Source: CAD feature listing. Evaluate the final solid. Frame: model axes, mm. A direction names the side the tool comes from. Give positions to 0.01 mm unless a question says otherwise; leave off trailing zeros. Loops run counter-clockwise (first coordinate to the right, second up) from the corner with the lowest first, then second, coordinate; pieces in that order, holes last. Notation, with made-up numbers: (46, -6.5) - (104, -6.5) arc R12 cw to (104, 13.5) - close; hole circle Ø6 at (38.5, -28). An arc over 180 degrees is marked (long way). Write each question's results on one line, items separated by ' | '. Start each with the question number.
(1) Contact query for flat-ended pins moving along their axis: pin 1 (1.5 mm diameter, centred on y = 4.5, z = 0, fed in from -X); pin 2 (1 mm diameter, centred on x = 43.5, z = -0.5, fed in from -Y); pin 3 (5 mm diameter, centred on x = 76, y = 3, fed in from -Z). Output: stop coordinate, or through.
(2) Reachability of faces 4 (the cylindrical face through (152.449, 2.385, 1.197)), 5 (the cylindrical face through (-0.97, -0.92, 1.81)) from +Z, -Z, +X, -X, +Y, -Y: full face, straight path, thin tool, end or side. Return the list, or none.
(3) Cut plane A-A on x = 9. Return the cut outline in (y, z), then the cut area to 3 significant figures.
(4) Material intervals for line 1 along Y through (x, z) = (65, -0.3); line 2 along Y through (x, z) = (54.5, -0.4); line 3 along X through (y, z) = (3.25, 0.65), sorted ascending. Write a range as [from, to].
(5) Pull-direction query (X, two-part tool) for faces 1 (the cylindrical face through (155.92, 10.97, 1.81)), 2 (the cylindrical face through (-0.97, 10.92, 1.81)), 3 (the cylindrical face through (2.551, 7.615, 1.197)); classes: pulls with the +X half, pulls with the -X half, needs draft (parallel to the pull), parting line crosses it, or undercut.
from build123d import *

# Parameters (mm, degrees)
F0_W         = 155
F0_H         = 10
F0_W_2       = 152.0637926605
F0_H_2       = 7.2836262298
F1_DEPTH     = 1.2
F2_W         = 159
F2_H         = 14
F2_W_2       = 155
F2_H_2       = 10
F2_W_3       = 152.0637926605
F2_H_3       = 7.2836262298
F3_DEPTH     = 1.2
F4_W         = 155
F4_H         = 1
F5_DEPTH     = 1.2
F6_R         = 3.6
F7_T1_DEPTH  = 160
F7_T3_DEPTH  = 0.0836262298
F7_T5_DEPTH  = 144.8637926605
F7_T10_ANGLE = 129.8047192326
F7_T13_ANGLE = 90
F7_T17_ANGLE = 129.8047192326
F7_T22_ANGLE = 129.8047192326
F7_T25_ANGLE = 90
F7_T27_ANGLE = 90
F7_T29_ANGLE = 90
F7_T33_ANGLE = 129.8047192326
F8_F1_R      = 0.5
F8_F2_R      = 0.5
F8_F3_R      = 0.5


# Not quite as in the source:
# - a fillet or chamfer that OpenCascade refuses, or shapes differently, is made with other operations: its cross-section is extruded or revolved along the edge and cut away or added


with BuildPart() as f1:
    # F0 (on Top) → F1 (new body)
    with BuildSketch(Plane.XY):
        with Locations((77.5, 5)):
            Rectangle(F0_W, F0_H)
        with Locations((77.5, 5)):
            Rectangle(F0_W_2, F0_H_2, mode=Mode.SUBTRACT)
    extrude(amount=F1_DEPTH)

    # F2 (on face) → F3 (join)
    with BuildSketch(Plane.XY.offset(1.2)):
        with Locations((77.5, 5)):
            Rectangle(F2_W, F2_H)
        with Locations((77.5, 5)):
            Rectangle(F2_W_2, F2_H_2, mode=Mode.SUBTRACT)
        with Locations((77.5, 5)):
            Rectangle(F2_W_2, F2_H_2)
        with Locations((77.5, 5)):
            Rectangle(F2_W_3, F2_H_3, mode=Mode.SUBTRACT)
    extrude(amount=F3_DEPTH)

    # F4 (on face) → F5 (join)
    with BuildSketch(Plane(origin=(0, 0, 0), x_dir=(1, 0, 0), z_dir=(0, 0, -1))):
        with Locations((77.5, 0.5)):
            Rectangle(F4_W, F4_H)
        Polygon((155, -1.3581868851), (155, 0), (0, 0), (0, -1.3581868851), (1.4681036697, -1.3581868851), (153.5318963303, -1.3581868851), align=None)
        Polygon((155, -10), (155, -8.6418131149), (153.5318963303, -8.6418131149), (1.4681036697, -8.6418131149), (0, -8.6418131149), (0, -10), align=None)
        with Locations((77.5, -10.5)):
            Rectangle(F4_W, F4_H)
    extrude(amount=F5_DEPTH)

    # F6
    f6_edges = [f1.edges().sort_by_distance(p)[0] for p in [
        (1.468104, 1.358187, 1.2),
        (1.468104, 8.641813, 1.2),
        (153.531896, 1.358187, 1.2),
        (153.531896, 8.641813, 1.2),
        (157, -2, 1.8),
        (157, 12, 1.8),
        (-2, 12, 1.8),
        (-2, -2, 1.8),
    ]]
    fillet(f6_edges, radius=F6_R)

    # F7: fillet of radius 1 on 16 edges, made by hand

    # F7_s2 → F7_t1 (cut)
    with BuildSketch(Plane.YZ.offset(-2.5)):
        with BuildLine():
            ThreePointArc((1.3581868851, -0.2), (1.0652936663, -0.9071067812), (0.3581868851, -1.2))
            Line((0.3581868851, -1.2), (1.3581868851, -1.2))
            Line((1.3581868851, -1.2), (1.3581868851, -0.2))
        make_face()
        with BuildLine():
            ThreePointArc((8.6418131149, -0.2), (8.9347063337, -0.9071067812), (9.6418131149, -1.2))
            Line((9.6418131149, -1.2), (8.6418131149, -1.2))
            Line((8.6418131149, -1.2), (8.6418131149, -0.2))
        make_face()
    extrude(amount=F7_T1_DEPTH, mode=Mode.SUBTRACT)

    # F7_s4 → F7_t3 (cut)
    with BuildSketch(Plane.XZ.offset(-5.0418131149)):
        with BuildLine():
            ThreePointArc((0.4681036697, 0), (1.1752104509, 0.2928932188), (1.4681036697, 1))
            Line((1.4681036697, 1), (1.4681036697, 0))
            Line((1.4681036697, 0), (0.4681036697, 0))
        make_face()
        with BuildLine():
            ThreePointArc((1.4681036697, 1.4), (1.1752104509, 2.1071067812), (0.4681036697, 2.4))
            Line((0.4681036697, 2.4), (1.4681036697, 2.4))
            Line((1.4681036697, 2.4), (1.4681036697, 1.4))
        make_face()
        with BuildLine():
            ThreePointArc((154.5318963303, 2.4), (153.8247895491, 2.1071067812), (153.5318963303, 1.4))
            Line((153.5318963303, 1.4), (153.5318963303, 2.4))
            Line((153.5318963303, 2.4), (154.5318963303, 2.4))
        make_face()
        with BuildLine():
            ThreePointArc((154.5318963303, 0), (153.8247895491, 0.2928932188), (153.5318963303, 1))
            Line((153.5318963303, 1), (153.5318963303, 0))
            Line((153.5318963303, 0), (154.5318963303, 0))
        make_face()
    extrude(amount=F7_T3_DEPTH, mode=Mode.SUBTRACT)

    # F7_s6 → F7_t5 (cut)
    with BuildSketch(Plane.YZ.offset(5.0681036697)):
        with BuildLine():
            ThreePointArc((1.3581868851, 1.4), (1.0652936663, 2.1071067812), (0.3581868851, 2.4))
            Line((0.3581868851, 2.4), (1.3581868851, 2.4))
            Line((1.3581868851, 2.4), (1.3581868851, 1.4))
        make_face()
        with BuildLine():
            ThreePointArc((8.6418131149, 1.4), (8.9347063337, 2.1071067812), (9.6418131149, 2.4))
            Line((9.6418131149, 2.4), (8.6418131149, 2.4))
            Line((8.6418131149, 2.4), (8.6418131149, 1.4))
        make_face()
    extrude(amount=F7_T5_DEPTH, mode=Mode.SUBTRACT)


with BuildPart() as f7_tool8:
    # F7_s9 → F7_t10 (revolve)
    with BuildSketch(Plane(origin=(0.5115194158, -0.4262532935, 0), x_dir=(0, 0, 1), z_dir=(0.7682307976, -0.6401729779, 0))):
        with BuildLine():
            ThreePointArc((0, -11.7177391291), (0.2928932188, -11.0106323479), (1, -10.7177391291))
            Line((1, -10.7177391291), (0, -10.7177391291))
            Line((0, -10.7177391291), (0, -11.7177391291))
        make_face()
    revolve(axis=Axis((5.0681036697, 5.0418131149, 0), (0, 0, 1)), revolution_arc=F7_T10_ANGLE)

    split(bisect_by=Plane.XZ.offset(-8.6418131149), keep=Keep.TOP)


with BuildPart() as f1_1:
    add(f1.part)

    # F7_t7: cut F7_tool8
    add(f7_tool8.part, mode=Mode.SUBTRACT)

    # F7_s12 → F7_t13 (revolve, cut)
    with BuildSketch(Plane.YZ.offset(5.0681036697)):
        with BuildLine():
            ThreePointArc((8.6418131149, 1.4), (8.9347063337, 2.1071067812), (9.6418131149, 2.4))
            Line((9.6418131149, 2.4), (8.6418131149, 2.4))
            Line((8.6418131149, 2.4), (8.6418131149, 1.4))
        make_face()
    revolve(axis=Axis((5.0681036697, 5.0418131149, 2.4), (0, 0, 1)), revolution_arc=F7_T13_ANGLE, mode=Mode.SUBTRACT)


with BuildPart() as f7_tool15:
    # F7_s16 → F7_t17 (revolve)
    with BuildSketch(Plane(origin=(90.9661571375, 75.8028393036, 0), x_dir=(0, 0, 1), z_dir=(-0.7682307976, -0.6401729779, 0))):
        with BuildLine():
            ThreePointArc((0, -87.5090724404), (0.2928932188, -88.2161792216), (1, -88.5090724404))
            Line((1, -88.5090724404), (0, -88.5090724404))
            Line((0, -88.5090724404), (0, -87.5090724404))
        make_face()
    revolve(axis=Axis((149.9318963303, 5.0418131149, 0), (0, 0, -1)), revolution_arc=F7_T17_ANGLE)

    split(bisect_by=Plane.XZ.offset(-8.6418131149), keep=Keep.TOP)


with BuildPart() as f1_2:
    add(f1_1.part)

    # F7_t14: cut F7_tool15
    add(f7_tool15.part, mode=Mode.SUBTRACT)


with BuildPart() as f7_tool20:
    # F7_s21 → F7_t22 (revolve)
    with BuildSketch(Plane.XZ.offset(-4.9581868851)):
        with BuildLine():
            ThreePointArc((0.4681036697, 0), (1.1752104509, 0.2928932188), (1.4681036697, 1))
            Line((1.4681036697, 1), (1.4681036697, 0))
            Line((1.4681036697, 0), (0.4681036697, 0))
        make_face()
    revolve(axis=Axis((5.0681036697, 4.9581868851, 0), (0, 0, 1)), revolution_arc=F7_T22_ANGLE)

    split(bisect_by=Plane.XZ.offset(-1.3581868851), keep=Keep.BOTTOM)


with BuildPart() as f1_3:
    add(f1_2.part)

    # F7_t19: cut F7_tool20
    add(f7_tool20.part, mode=Mode.SUBTRACT)

    # F7_s24 → F7_t25 (revolve, cut)
    with BuildSketch(Plane.XZ.offset(-4.9581868851)):
        with BuildLine():
            ThreePointArc((1.4681036697, 1.4), (1.1752104509, 2.1071067812), (0.4681036697, 2.4))
            Line((0.4681036697, 2.4), (1.4681036697, 2.4))
            Line((1.4681036697, 2.4), (1.4681036697, 1.4))
        make_face()
    revolve(axis=Axis((5.0681036697, 4.9581868851, 2.4), (0, 0, 1)), revolution_arc=F7_T25_ANGLE, mode=Mode.SUBTRACT)

    # F7_s26 → F7_t27 (revolve, cut)
    with BuildSketch(Plane.YZ.offset(149.9318963303)):
        with BuildLine():
            ThreePointArc((9.6418131149, 2.4), (8.9347063337, 2.1071067812), (8.6418131149, 1.4))
            Line((8.6418131149, 1.4), (8.6418131149, 2.4))
            Line((8.6418131149, 2.4), (9.6418131149, 2.4))
        make_face()
    revolve(axis=Axis((149.9318963303, 5.0418131149, 2.4), (0, 0, -1)), revolution_arc=F7_T27_ANGLE, mode=Mode.SUBTRACT)

    # F7_s28 → F7_t29 (revolve, cut)
    with BuildSketch(Plane.YZ.offset(149.9318963303)):
        with BuildLine():
            ThreePointArc((0.3581868851, 2.4), (1.0652936663, 2.1071067812), (1.3581868851, 1.4))
            Line((1.3581868851, 1.4), (1.3581868851, 2.4))
            Line((1.3581868851, 2.4), (0.3581868851, 2.4))
        make_face()
    revolve(axis=Axis((149.9318963303, 4.9581868851, 2.4), (0, 0, 1)), revolution_arc=F7_T29_ANGLE, mode=Mode.SUBTRACT)


with BuildPart() as f7_tool31:
    # F7_s32 → F7_t33 (revolve)
    with BuildSketch(Plane(origin=(86.0481511635, -71.7046248877, 0), x_dir=(0, 0, 1), z_dir=(-0.7682307976, 0.6401729779, 0))):
        with BuildLine():
            ThreePointArc((1, 96.1913804165), (0.2928932188, 95.8984871977), (0, 95.1913804165))
            Line((0, 95.1913804165), (0, 96.1913804165))
            Line((0, 96.1913804165), (1, 96.1913804165))
        make_face()
    revolve(axis=Axis((149.9318963303, 4.9581868851, 0), (0, 0, 1)), revolution_arc=F7_T33_ANGLE)

    split(bisect_by=Plane.XZ.offset(-1.3581868851), keep=Keep.BOTTOM)


with BuildPart() as f1_4:
    add(f1_3.part)

    # F7_t30: cut F7_tool31
    add(f7_tool31.part, mode=Mode.SUBTRACT)

    # F8: fillet of radius 0.5 on 10 edges, made by hand

    # F8_f1
    f8_f1_edges = [f1_4.edges().sort_by_distance(p)[0] for p in [
        (77.5, 0, 0),
        (77.5, 10, 0),
    ]]
    fillet(f8_f1_edges, radius=F8_F1_R)

    # F8_f2
    f8_f2_edges = [f1_4.edges().sort_by_distance(p)[0] for p in [
        (0, 0, 0.85),
        (155, 0, 0.85),
        (155, 10, 0.85),
        (0, 10, 0.85),
        (0, 10.1464466094, 0.1464466094),
        (155, 10.1464466094, 0.1464466094),
        (155, -0.1464466094, 0.1464466094),
        (0, -0.1464466094, 0.1464466094),
    ]]
    fillet(f8_f2_edges, radius=F8_F2_R)

    # F8_f3
    f8_f3_edges = [f1_4.edges().sort_by_distance(p)[0] for p in [
        (77.5, 0, 1.2),
        (77.5, 10, 1.2),
        (155, 5, 1.2),
        (0, 5, 1.2),
        (0.1464466094, 9.8535533906, 1.2),
        (0.1464466094, 0.1464466094, 1.2),
        (154.8535533906, 0.1464466094, 1.2),
        (154.8535533906, 9.8535533906, 1.2),
    ]]
    fillet(f8_f3_edges, radius=F8_F3_R)


solid = f1_4.part
Ans:
1) pin 1: x = 0 | pin 2: y = -1 | pin 3: z = -1.19
2) face 4: +Z, -Z | face 5: +Z, -Z, -X, -Y
3) outline: (-2, 1.2) - (-0.5, 1.2) arc R0.5 cw to (0, 0.7) - (0, 0.5) arc R0.5 cw to (-0.5, 0) - (-1, 0) - (-1, -1.2) - (0.36, -1.2) arc R1 ccw to (1.36, -0.2) - (1.36, 1.4) arc R1 ccw to (0.36, 2.4) - (-2, 2.4) - close; (8.64, -0.2) arc R1 ccw to (9.64, -1.2) - (11, -1.2) - (11, 0) - (10.5, 0) arc R0.5 cw to (10, 0.5) - (10, 0.7) arc R0.5 cw to (10.5, 1.2) - (12, 1.2) - (12, 2.4) - (9.64, 2.4) arc R1 ccw to (8.64, 1.4) - close | area: 16.3 mm^2
4) line 1: [-1, 1.35], [8.65, 11] | line 2: [-1, 1.34], [8.66, 11] | line 3: [0, 1.83], [153.17, 155]
5) face 1: pulls with the +X half | face 2: pulls with the -X half | face 3: undercut
